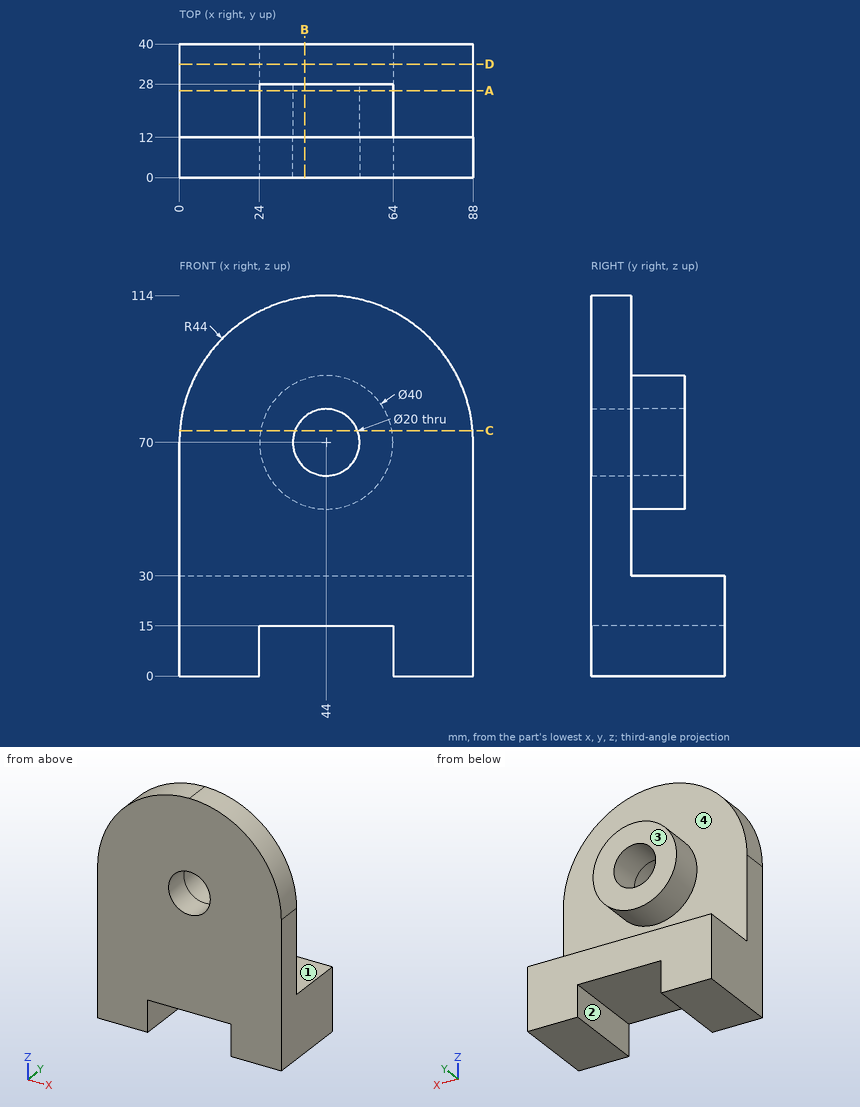
Print and shaded views of the part. All mm, measured from the part's lowest x, y and z. A direction names the side the tool comes from. Coordinates: 2 decimals unless noted, no trailing zeros. Order: outer loops, then holes, each group sorted by start corner. A loop starts at its lowest first (then second) coordinate and runs counter-clockwise, first axis right, second up. Notation, with made-up numbers: (43, 3.5) -> (78, 3.5) arc R9 ccw to (78, 19.5) -> close; hole circle Ø5 at (65.5, 77.5). An arc over 180 degrees is marked (long way). Use one line per item in the form item = value. Start each with the question number.
1) Band-saw the part on C-C on z = 73.5. Give the cut face in (x, y).
2) Drill centre lines: L1, parallel to Z at x = 44, y = 23; L2, parallel to Z at x = 44, y = 8; L3, parallel to Y at x = 34.5, z = 59.5. Where is each one in solid material? Low to high. Write a range as [from, to].
3) Drop flat-ended pins along their axis: pin 1 (12 mm diameter, centred on x = 71, z = 30.5, fed in from +Y); pin 2 (12 mm diameter, centred on x = 10.5, y = 30, fed in from +Z); pin 3 (2 mm diameter, centred on y = 8, z = 78, fed in from +X); pin 4 (14 mm diameter, centred on x = 44.5, y = 21.5, fed in from +Z). Give the stop position or say it passes through.
4) Band-saw the part on D-D on y = 34. Give the cut face in (x, z), then the cut area to 3 significant figures.
5) Tool access for the marked faces 1, 2, 3 and 4: list every direction of +Z, -Z, +X, -X, +Y, -Y with a clear straight run to the whole face (end or side of a thin tool).
6) Band-saw the part on B-B on x = 37.5. Give the cut face in (y, z), then the cut area to 3 significant figures.
7) Band-saw the part on A-A on y = 26. Give the cut face in (x, z).
Entries:
q1.outline = (0.14, 0) -> (34.63, 0) -> (34.63, 28) -> (24.31, 28) -> (24.31, 12) -> (0.14, 12) -> close; (53.37, 0) -> (87.86, 0) -> (87.86, 12) -> (63.69, 12) -> (63.69, 28) -> (53.37, 28) -> close
q2.L1 = [15, 30], [50, 60], [80, 90]
q2.L2 = [15, 60], [80, 114]
q2.L3 = [0, 28]
q3.pin_1 = 40
q3.pin_2 = 30
q3.pin_3 = 87.44
q3.pin_4 = 90
q4.outline = (0, 0) -> (24, 0) -> (24, 15) -> (64, 15) -> (64, 0) -> (88, 0) -> (88, 30) -> (0, 30) -> close
q4.area = 2,040 mm2
q5.face_1 = +X, -X, +Y
q5.face_2 = -Z, +Y, -Y
q5.face_3 = +Z, +X, -X, +Y
q5.face_4 = +Y
q6.outline = (0, 15) -> (40, 15) -> (40, 30) -> (12, 30) -> (12, 51.09) -> (28, 51.09) -> (28, 62.4) -> (0, 62.4) -> close; (0, 77.6) -> (28, 77.6) -> (28, 88.91) -> (12, 88.91) -> (12, 113.52) -> (0, 113.52) -> close
q6.area = 1,780 mm2
q7.outline = (0, 0) -> (24, 0) -> (24, 15) -> (64, 15) -> (64, 0) -> (88, 0) -> (88, 30) -> (0, 30) -> close; circle Ø40 at (44, 70); hole circle Ø20 at (44, 70)
